```python
from build123d import *

# Parameters (mm, degrees)
SKETCH1_W           = 46
SKETCH1_H           = 54
SKETCH1_R           = 2.45
SKETCH1_R_2         = 1.45
BOSS_EXTRUDE1_DEPTH = 0.6
SKETCH1_3_R         = 2.45
SKETCH1_3_R_2       = 1.45
BOSS_EXTRUDE2_DEPTH = 2
FILLET1_R           = 5


with BuildPart() as part:
    # Sketch1 → Boss-Extrude1 (new body)
    with BuildSketch(Plane(origin=(0, 0, 0), x_dir=(1, 0, 0), z_dir=(0, 1, 0))):
        Rectangle(SKETCH1_W, SKETCH1_H)
        with Locations((19, -23)):
            Circle(SKETCH1_R, mode=Mode.SUBTRACT)
        with Locations((-19, -23)):
            Circle(SKETCH1_R, mode=Mode.SUBTRACT)
        with Locations((19, 23)):
            Circle(SKETCH1_R, mode=Mode.SUBTRACT)
        with Locations((-19, 23)):
            Circle(SKETCH1_R, mode=Mode.SUBTRACT)
        with Locations((-19, 23)):
            Circle(SKETCH1_R)
        with Locations((-19, 23)):
            Circle(SKETCH1_R_2, mode=Mode.SUBTRACT)
        with Locations((19, 23)):
            Circle(SKETCH1_R)
        with Locations((19, 23)):
            Circle(SKETCH1_R_2, mode=Mode.SUBTRACT)
        with Locations((-19, -23)):
            Circle(SKETCH1_R)
        with Locations((-19, -23)):
            Circle(SKETCH1_R_2, mode=Mode.SUBTRACT)
        with Locations((19, -23)):
            Circle(SKETCH1_R)
        with Locations((19, -23)):
            Circle(SKETCH1_R_2, mode=Mode.SUBTRACT)
    extrude(amount=BOSS_EXTRUDE1_DEPTH)

    # Sketch1_3 → Boss-Extrude2 (add)
    with BuildSketch(Plane(origin=(0, 0, 0), x_dir=(1, 0, 0), z_dir=(0, 1, 0))):
        with Locations((-19, -23)):
            Circle(SKETCH1_3_R)
        with Locations((-19, -23)):
            Circle(SKETCH1_3_R_2, mode=Mode.SUBTRACT)
        with Locations((19, -23)):
            Circle(SKETCH1_3_R)
        with Locations((19, -23)):
            Circle(SKETCH1_3_R_2, mode=Mode.SUBTRACT)
        with Locations((-19, 23)):
            Circle(SKETCH1_3_R)
        with Locations((-19, 23)):
            Circle(SKETCH1_3_R_2, mode=Mode.SUBTRACT)
        with Locations((19, 23)):
            Circle(SKETCH1_3_R)
        with Locations((19, 23)):
            Circle(SKETCH1_3_R_2, mode=Mode.SUBTRACT)
    extrude(amount=BOSS_EXTRUDE2_DEPTH)

    # Fillet1
    fillet1_edges = [part.edges().sort_by_distance(p)[0] for p in [
        (23, 0.3, -27),
        (23, 0.3, 27),
        (-23, 0.3, 27),
        (-23, 0.3, -27),
    ]]
    fillet(fillet1_edges, radius=FILLET1_R)


solid = part.part
```
Source: CAD feature listing. Evaluate the final solid. Frame: model axes, mm. A direction names the side the tool comes from. Give positions to 0.01 mm unless a question says otherwise; leave off trailing zeros. Order: outer loops, then holes, each group sorted by start corner. A loop starts at its lowest first (then second) coordinate and runs counter-clockwise, first axis right, second up. Notation, with made-up numbers: (-32, 58) -> (-22, 58) arc R21 cw to (-22, 77) -> close; hole circle Ø5 at (65.5, -39). An arc over 180 degrees is marked (long way). Use a Markdown table: item, result.
Q1. Access query for faces 4 (the face through (16.552, 1.29, -23.108)), 5 (the face through (21.5, 0.3, -25.57)). Directions: +Z, -Z, +X, -X, +Y, -Y. A direction counts if a zero-diameter tool reaches every point of the face in a straight line with its end or side. Return the directions, or none.
A:
| item | result |
|---|---|
| face 4 | +Y |
| face 5 | -Z, +X, +Y, -Y |
Q2. Section B-B (z = -23). Return the cut outline in (x, y).
A:
| item | result |
|---|---|
| outline | (-22.9, 0) -> (-20.45, 0) -> (-20.45, 2) -> (-21.45, 2) -> (-21.45, 0.6) -> (-22.9, 0.6) -> close; (-17.55, 0) -> (17.55, 0) -> (17.55, 2) -> (16.55, 2) -> (16.55, 0.6) -> (-16.55, 0.6) -> (-16.55, 2) -> (-17.55, 2) -> close; (20.45, 0) -> (22.9, 0) -> (22.9, 0.6) -> (21.45, 0.6) -> (21.45, 2) -> (20.45, 2) -> close |
Q3. First-contact query: P1, Ø1.7, axis at x = -19, z = -23, coming from the -Y side; P2, Ø1.5, axis at x = -1, z = -14.5, coming from the +Y side. Flat tips, straight axial feed; report the tip coordinate or a pass-through.
A:
| item | result |
|---|---|
| P1 | through |
| P2 | y = 0.6 |
Q4. Pull-direction query (X, two-part tool) for faces 1 (the face through (-21.5, 0.3, -25.57)), 2 (the face through (19, 2, 25)), 3 (the face through (20.339, 0.986, -22.445)); classes: +X half, -X half, draft (parallel to the pull), parting line (faces both ways), or undercut.
A:
| item | result |
|---|---|
| face 1 | -X half |
| face 2 | draft |
| face 3 | undercut |
Q5. Section D-D (x = 10). Return the cut outline in (y, z).
A:
| item | result |
|---|---|
| outline | (0, -27) -> (0.6, -27) -> (0.6, 27) -> (0, 27) -> close |
Q6. Material intervals for line 1 (X direction, y = 1.15, z = 23); line 2 (Z direction, x = 19, y = 1); line 3 (Y direction, x = 8.5, z = 8), sorted ascending. Write a range as [from, to].
A:
| item | result |
|---|---|
| line 1 | [-21.45, -20.45], [-17.55, -16.55], [16.55, 17.55], [20.45, 21.45] |
| line 2 | [-25.45, -24.45], [-21.55, -20.55], [20.55, 21.55], [24.45, 25.45] |
| line 3 | [0, 0.6] |
Q7. Section A-A (y = 1.3). Return the cut outline in (x, z).
A:
| item | result |
|---|---|
| outline | circle Ø4.9 at (-19, -23); circle Ø4.9 at (-19, 23); circle Ø4.9 at (19, -23); circle Ø4.9 at (19, 23); hole circle Ø2.9 at (-19, -23); hole circle Ø2.9 at (-19, 23); hole circle Ø2.9 at (19, -23); hole circle Ø2.9 at (19, 23) |
Q8. Section C-C (x = 19). Return the cut outline in (y, z), and give its area (3 significant figures).
A:
| item | result |
|---|---|
| outline | (0, -26.9) -> (0.6, -26.9) -> (0.6, -25.45) -> (2, -25.45) -> (2, -24.45) -> (0, -24.45) -> close; (0, -21.55) -> (2, -21.55) -> (2, -20.55) -> (0.6, -20.55) -> (0.6, 20.55) -> (2, 20.55) -> (2, 21.55) -> (0, 21.55) -> close; (0, 24.45) -> (2, 24.45) -> (2, 25.45) -> (0.6, 25.45) -> (0.6, 26.9) -> (0, 26.9) -> close |
| area | 34.4 mm^2 |
